```python
from build123d import *

# Parameters (mm, degrees)
BASPROSKE_W        = 8
BASPROSKE_H        = 16.5
TOOTHCUT_DEPTH     = 25.667792767
TEETHCUTS_COUNT    = 20
TEETHCUTS_ANGLE    = 342
BORSKE_R           = 0.4
BORE_DEPTH         = 50.0000508
CUT_EXTRUDE1_DEPTH = 25.496234031


with BuildPart() as part:
    # BasProSke → Base-Revolve (revolve)
    with BuildSketch(Plane(origin=(0, 0, 0), x_dir=(1, 0, 0), z_dir=(0, 1, 0)), mode=Mode.PRIVATE) as base_revolve_sk:
        with Locations((4, 8.25)):
            Rectangle(BASPROSKE_W, BASPROSKE_H)
    revolve(base_revolve_sk.sketch.rotate(Axis((-10, 0, 0), (1, 0, 0)), 180), axis=Axis((-10, 0, 0), (1, 0, 0)))

    # TooCutSke → ToothCut (cut, through all)
    with BuildSketch(Plane(origin=(0, 0, 0), x_dir=(0, 0, -1), z_dir=(1, 0, 0))):
        with BuildLine():
            ThreePointArc((0.877929023, 13.094602576), (0, 13.124), (-0.877929023, 13.094602576))
            ThreePointArc((-0.877929023, 13.094602576), (-1.227785764, 14.834041313), (-2.071065599, 16.395106966))
            ThreePointArc((-2.071065599, 16.395106966), (0, 16.5254), (2.071065599, 16.395106966))
            ThreePointArc((2.071065599, 16.395106966), (1.227785764, 14.834041313), (0.877929023, 13.094602576))
        make_face()
    toothcut = extrude(amount=TOOTHCUT_DEPTH, mode=Mode.SUBTRACT)

    # TeethCuts: ToothCut ×20 about axis
    teethcuts_axis = Axis((-10, 0, 0), (1, 0, 0))
    for i in range(1, TEETHCUTS_COUNT):
        add(toothcut.rotate(teethcuts_axis, i * TEETHCUTS_ANGLE / (TEETHCUTS_COUNT - 1)), mode=Mode.SUBTRACT)

    # BorSke → Bore (cut, symmetric)
    with BuildSketch(Plane(origin=(0, 0, 0), x_dir=(0, 0, -1), z_dir=(1, 0, 0))):
        with Locations(Location((0, 0, 0), (0, 0, 180))):
            Circle(BORSKE_R)
    extrude(amount=BORE_DEPTH, both=True, mode=Mode.SUBTRACT)

    # Sketch1 → Cut-Extrude1 (cut, through all)
    with BuildSketch(Plane(origin=(8, 0, 0), x_dir=(0, 0, -1), z_dir=(1, 0, 0))):
        with BuildLine():
            ThreePointArc((2, 0), (1.8851176, 0.668080559), (1.553668367, 1.25941042))
            Line((1.553668367, 1.25941042), (-1.553668367, 1.25941042))
            ThreePointArc((-1.553668367, 1.25941042), (-0.668080559, -1.8851176), (2, 0))
        make_face()
    extrude(amount=-CUT_EXTRUDE1_DEPTH, mode=Mode.SUBTRACT)


solid = part.part
```
Work out the finished part from the listing and answer in its coordinate system (mm). A direction names the side the tool comes from. Coordinates: 2 decimals unless noted, no trailing zeros. Loops run counter-clockwise (first coordinate to the right, second up) from the corner with the lowest first, then second, coordinate; pieces in that order, holes last. Notation, with made-up numbers: (70, 50) -> (84, 50) arc R25 cw to (84, 88) -> close; hole circle Ø1 at (-32, -33.75). An arc over 180 degrees is marked (long way). Answer as CSV lines item,"result".
Q1. The part is cut by section B-B on y = 13.5. Write down the section's boundary in (x, z), and give its area (3 significant figures).
Findings:
outline,"(0, -7.9) -> (8, -7.9) -> (8, -5.58) -> (0, -5.58) -> close; (0, -3.37) -> (8, -3.37) -> (8, -0.91) -> (0, -0.91) -> close; (0, 0.91) -> (8, 0.91) -> (8, 3.37) -> (0, 3.37) -> close; (0, 5.58) -> (8, 5.58) -> (8, 7.9) -> (0, 7.9) -> close"
area,"76.3 mm²"
Q2. Find the intervals of material crossed by probe 1 along Y at (x, z) = (6, 0); probe 2 along Y at (x, z) = (1.25, 11.5); probe 3 along Z at (x, y) = (3.5, -7.5), in increasing order.
Findings:
probe 1,"y = -13.12 to -2, 1.26 to 13.12"
probe 2,"y = -11.83 to -10.06, -7.22 to 7.22, 10.06 to 11.83"
probe 3,"z = -14.7 to -12.08, -10.77 to 10.77, 12.08 to 14.7"
Q3. A tool of negligible diameter and unlimited length cuts with its end or side. For faces 5 (the face through (3.944, 0.012, 13.124)), 6 (the face through (3.944, 11.285, -9.721)), 7 (the face through (3.944, 14.498, 3.416)), from which of +Z, -Z, +X, -X, +Y, -Y can it reach the whole face along a straight path? Write none if from no direction.
Findings:
face 5,"+Z, +X, -X"
face 6,"+X, -X, +Y"
face 7,"+X, -X"
Q4. Each of these flat-tipped pins is pushed along its axis until it touches: pin 1 (4 mm diameter, centred on x = 2.5, z = -12, fed in from -Y); pin 2 (1.5 mm diameter, centred on x = 6.5, y = -12.5, fed in from -Z). Where does it stop, or does it pass through?
Findings:
pin 1,"stops at y = -12.04"
pin 2,"stops at z = -11.58"
Q5. For a pull along Y with two mould halves and no side action, classify faces 1 (the face through (3.94, -14.84, 1.23)), 2 (the face through (4.056, 7.484, -14.705)), 3 (the face through (3.944, 4.067, 12.478)), 4 (the face through (3.94, 1.23, 14.84)) as +Y half, -Y half, draft (parallel to the pull), parting line (faces both ways), or undercut.
Findings:
face 1,"-Y half"
face 2,"+Y half"
face 3,"undercut"
face 4,"undercut"
Q6. The part is cut by section D-D on z = 6. Write down the section's boundary in (x, y), and give its area (3 significant figures).
Findings:
outline,"(0, -14.03) -> (8, -14.03) -> (8, 14.03) -> (0, 14.03) -> close"
area,"224 mm²"
Q7. The part is cut by section A-A on z = 0. Write down the section's boundary in (x, y).
Findings:
outline,"(0, -13.12) -> (8, -13.12) -> (8, -2) -> (0, -2) -> close; (0, 1.26) -> (8, 1.26) -> (8, 13.12) -> (0, 13.12) -> close"
Q8. The part is cut by section C-C on z = -14. Write down the section's boundary in (x, y), and give its area (3 significant figures).
Findings:
outline,"(0, -7.95) -> (8, -7.95) -> (8, -5.98) -> (0, -5.98) -> close; (0, -3.41) -> (8, -3.41) -> (8, -0.99) -> (0, -0.99) -> close; (0, 0.99) -> (8, 0.99) -> (8, 3.41) -> (0, 3.41) -> close; (0, 5.98) -> (8, 5.98) -> (8, 7.95) -> (0, 7.95) -> close"
area,"70.3 mm²"
